from build123d import *

# Parameters (mm, degrees)
CROQUIS1_R              = 7.5
SALIENTE_EXTRUIR2_DEPTH = 20
SALIENTE_EXTRUIR3_DEPTH = 30
SALIENTE_EXTRUIR4_DEPTH = 80
CROQUIS4_R              = 10
CORTAR_EXTRUIR1_DEPTH   = 141.528466867


with BuildPart() as part:
    # Croquis1 → Saliente-Extruir2 (new body)
    # profile 1 of 7: a face of its own
    with BuildSketch(Plane(origin=(0, 0, 0), x_dir=(1, 0, 0), z_dir=(0, 1, 0))):
        with BuildLine():
            Line((74.169014085, 14.661423864), (6.338028169, 29.322847729))
            ThreePointArc((6.338028169, 29.322847729), (15.924993338, 25.424291282), (23.616731357, 18.5))
            ThreePointArc((23.616731357, 18.5), (26.900316488, 13.280548665), (29.047375097, 7.5))
            ThreePointArc((29.047375097, 7.5), (29.760890888, 3.780128774), (30, 0))
            ThreePointArc((30, 0), (29.760890888, -3.780128774), (29.047375097, -7.5))
            ThreePointArc((29.047375097, -7.5), (26.900316488, -13.280548665), (23.616731357, -18.5))
            ThreePointArc((23.616731357, -18.5), (15.924993338, -25.424291282), (6.338028169, -29.322847729))
            Line((6.338028169, -29.322847729), (74.169014085, -14.661423864))
            ThreePointArc((74.169014085, -14.661423864), (86, 0), (74.169014085, 14.661423864))
        make_face()
        with Locations(Location((71, 0, 0), (0, 0, 270))):
            Circle(CROQUIS1_R, mode=Mode.SUBTRACT)
    # profile 2 of 7: a face of its own
    with BuildSketch(Plane(origin=(0, 0, 0), x_dir=(1, 0, 0), z_dir=(0, 1, 0))):
        with BuildLine():
            ThreePointArc((-29.047375097, -7.5), (-26.900316488, -13.280548665), (-23.616731357, -18.5))
            Line((-23.616731357, -18.5), (23.616731357, -18.5))
            ThreePointArc((23.616731357, -18.5), (26.900316488, -13.280548665), (29.047375097, -7.5))
            Line((29.047375097, -7.5), (-29.047375097, -7.5))
        make_face()
    # profile 3 of 7: a face of its own
    with BuildSketch(Plane(origin=(0, 0, 0), x_dir=(1, 0, 0), z_dir=(0, 1, 0))):
        with BuildLine():
            ThreePointArc((-23.616731357, -18.5), (-15.924993338, -25.424291282), (-6.338028169, -29.322847729))
            ThreePointArc((-6.338028169, -29.322847729), (0, -30), (6.338028169, -29.322847729))
            ThreePointArc((6.338028169, -29.322847729), (15.924993338, -25.424291282), (23.616731357, -18.5))
            Line((23.616731357, -18.5), (-23.616731357, -18.5))
        make_face()
    # profile 4 of 7: a face of its own
    with BuildSketch(Plane(origin=(0, 0, 0), x_dir=(1, 0, 0), z_dir=(0, 1, 0))):
        with BuildLine():
            Line((29.047375097, 7.5), (-29.047375097, 7.5))
            ThreePointArc((-29.047375097, 7.5), (-30, 0), (-29.047375097, -7.5))
            Line((-29.047375097, -7.5), (29.047375097, -7.5))
            ThreePointArc((29.047375097, -7.5), (29.760890888, -3.780128774), (30, 0))
            ThreePointArc((30, 0), (29.760890888, 3.780128774), (29.047375097, 7.5))
        make_face()
    # profile 5 of 7: a face of its own
    with BuildSketch(Plane(origin=(0, 0, 0), x_dir=(1, 0, 0), z_dir=(0, 1, 0))):
        with BuildLine():
            Line((23.616731357, 18.5), (-23.616731357, 18.5))
            ThreePointArc((-23.616731357, 18.5), (-26.900316488, 13.280548665), (-29.047375097, 7.5))
            Line((-29.047375097, 7.5), (29.047375097, 7.5))
            ThreePointArc((29.047375097, 7.5), (26.900316488, 13.280548665), (23.616731357, 18.5))
        make_face()
    # profile 6 of 7: a face of its own
    with BuildSketch(Plane(origin=(0, 0, 0), x_dir=(1, 0, 0), z_dir=(0, 1, 0))):
        with BuildLine():
            ThreePointArc((6.338028169, 29.322847729), (0, 30), (-6.338028169, 29.322847729))
            ThreePointArc((-6.338028169, 29.322847729), (-15.924993338, 25.424291282), (-23.616731357, 18.5))
            Line((-23.616731357, 18.5), (23.616731357, 18.5))
            ThreePointArc((23.616731357, 18.5), (15.924993338, 25.424291282), (6.338028169, 29.322847729))
        make_face()
    # profile 7 of 7: a face of its own
    with BuildSketch(Plane(origin=(0, 0, 0), x_dir=(1, 0, 0), z_dir=(0, 1, 0))):
        with BuildLine():
            Line((-6.338028169, 29.322847729), (-74.169014085, 14.661423864))
            ThreePointArc((-74.169014085, 14.661423864), (-86, 0), (-74.169014085, -14.661423864))
            Line((-74.169014085, -14.661423864), (-6.338028169, -29.322847729))
            ThreePointArc((-6.338028169, -29.322847729), (-15.924993338, -25.424291282), (-23.616731357, -18.5))
            ThreePointArc((-23.616731357, -18.5), (-26.900316488, -13.280548665), (-29.047375097, -7.5))
            ThreePointArc((-29.047375097, -7.5), (-30, 0), (-29.047375097, 7.5))
            ThreePointArc((-29.047375097, 7.5), (-26.900316488, 13.280548665), (-23.616731357, 18.5))
            ThreePointArc((-23.616731357, 18.5), (-15.924993338, 25.424291282), (-6.338028169, 29.322847729))
        make_face()
        with Locations(Location((-71, 0, 0), (0, 0, 270))):
            Circle(CROQUIS1_R, mode=Mode.SUBTRACT)
    extrude(amount=SALIENTE_EXTRUIR2_DEPTH)

    # Croquis2 → Saliente-Extruir3 (add)
    with BuildSketch(Plane(origin=(0, 20, 0), x_dir=(1, 0, 0), z_dir=(0, 1, 0))):
        with BuildLine():
            Line((-23.616731357, 18.5), (23.616731357, 18.5))
            ThreePointArc((23.616731357, 18.5), (0, 30), (-23.616731357, 18.5))
        make_face()
        with BuildLine():
            Line((-23.616731357, -18.5), (23.616731357, -18.5))
            ThreePointArc((23.616731357, -18.5), (0, -30), (-23.616731357, -18.5))
        make_face()
    extrude(amount=SALIENTE_EXTRUIR3_DEPTH)

    # Croquis3 → Saliente-Extruir4 (add)
    with BuildSketch(Plane(origin=(0, 20, 0), x_dir=(1, 0, 0), z_dir=(0, 1, 0))):
        with BuildLine():
            ThreePointArc((-23.616731357, 18.5), (-26.900316488, 13.280548665), (-29.047375097, 7.5))
            Line((-29.047375097, 7.5), (29.047375097, 7.5))
            ThreePointArc((29.047375097, 7.5), (26.900316488, 13.280548665), (23.616731357, 18.5))
            Line((23.616731357, 18.5), (-23.616731357, 18.5))
        make_face()
        with BuildLine():
            Line((-29.047375097, -7.5), (29.047375097, -7.5))
            ThreePointArc((29.047375097, -7.5), (26.900316391, -13.280548617), (23.616731357, -18.5))
            Line((23.616731357, -18.5), (-23.616731357, -18.5))
            ThreePointArc((-23.616731357, -18.5), (-26.900316488, -13.280548665), (-29.047375097, -7.5))
        make_face()
    extrude(amount=SALIENTE_EXTRUIR4_DEPTH)

    # Croquis4 → Cortar-Extruir1 (cut, through all)
    with BuildSketch(Plane.XY.offset(18.5)):
        with Locations((0, 76)):
            Circle(CROQUIS4_R)
    extrude(amount=-CORTAR_EXTRUIR1_DEPTH, mode=Mode.SUBTRACT)


solid = part.part
Input: part model. Units: mm. Frame: model coordinates. A direction names the side the tool comes from. Coordinates: 2 decimals unless noted, no trailing zeros. Order: outer loops, then holes, each group sorted by start corner. A loop starts at its lowest first (then second) coordinate and runs counter-clockwise, first axis right, second up. Notation, with made-up numbers: M -31.75,-4.75 L 9.25,-4.75 A25 cw 9.25,19.25 Z; hole C -7,37 d3. An arc over 180 degrees is marked long. Answer in a Markdown table with one row per item.
(1) Section query C-C, the plane y = 40.5. Output: boundary loops of the cut face in (x, z).
Numbers:
| item | result |
|---|---|
| outline | M -29.05,-7.5 A30 ccw 29.05,-7.5 Z; M -29.05,7.5 L 29.05,7.5 A30 ccw 23.62,18.5 A30 ccw Z |
(2) Draft query along X for faces 1 (the cylindrical face through (-77.654, 9.86, 3.461)), 2 (the flat face through (39.779, 9.86, 22.095)), 3 (the cylindrical face through (63.68, 9.86, -1.63)), 4 (the flat face through (0, 50, -23)). Return one class per face: pulls with the +X half, pulls with the -X half, needs draft (parallel to the pull), parting line crosses it, or undercut.
Numbers:
| item | result |
|---|---|
| face 1 | undercut |
| face 2 | pulls with the +X half |
| face 3 | undercut |
| face 4 | needs draft |
(3) Access query for faces 5 (the flat face through (0, 50, 23)), 6 (the flat face through (0, 100, -13)), 7 (the flat face through (0, 59, -7.5)). Directions: +Z, -Z, +X, -X, +Y, -Y. A direction counts if a zero-diameter tool reaches every point of the face in a straight line with its end or side. Return the directions, or none.
Numbers:
| item | result |
|---|---|
| face 5 | +Z, +X, -X, +Y |
| face 6 | +Z, -Z, +X, -X, +Y |
| face 7 | +X, -X, +Y |
(4) Material intervals for line 1 (X direction, y = 15, z = 0); line 2 (Y direction, x = -76, z = -6); line 3 (Z direction, x = -1, y = 30), sorted ascending. Write a range as [from, to].
Numbers:
| item | result |
|---|---|
| line 1 | x = [-86, -78.5], [-63.5, 63.5], [78.5, 86] |
| line 2 | y = [0, 20] |
| line 3 | z = [-29.98, -7.5], [7.5, 29.98] |
(5) Section query D-D, the plane x = 3.5. Output: boundary loops of the cut face in (y, z).
Numbers:
| item | result |
|---|---|
| outline | M 0,-29.8 L 50,-29.8 L 50,-18.5 L 66.63,-18.5 L 66.63,-7.5 L 20,-7.5 L 20,7.5 L 66.63,7.5 L 66.63,18.5 L 50,18.5 L 50,29.8 L 0,29.8 Z; M 85.37,-18.5 L 100,-18.5 L 100,-7.5 L 85.37,-7.5 Z; M 85.37,7.5 L 100,7.5 L 100,18.5 L 85.37,18.5 Z |
(6) Section query B-B, the plane y = 76. Output: boundary loops of the cut face in (x, z), plus the area to 3 significant figures.
Numbers:
| item | result |
|---|---|
| outline | M -29.05,-7.5 A30 ccw -23.62,-18.5 L -10,-18.5 L -10,-7.5 Z; M -29.05,7.5 L -10,7.5 L -10,18.5 L -23.62,18.5 A30 ccw Z; M 10,-18.5 L 23.62,-18.5 A30 ccw 29.05,-7.5 L 10,-7.5 Z; M 10,7.5 L 29.05,7.5 A30 ccw 23.62,18.5 L 10,18.5 Z |
| area | 739 mm^2 |
(7) Contact query for flat-ended pins moving along their axis: pin 1 Ø6 at (y, z) = (86, -16.5) entering from -X; pin 2 Ø4 at (y, z) = (73.5, 8.5) entering from -X; pin 3 Ø12 at (x, y) = (0, 76) entering from -Z; pin 4 Ø6 at (x, z) = (-10.5, 27) entering from +Y. Output: stop coordinate, or through.
Numbers:
| item | result |
|---|---|
| pin 1 | stops at x = -26.79 |
| pin 2 | stops at x = -29.05 |
| pin 3 | passes through |
| pin 4 | stops at y = 50 |
(8) Section query A-A, the plane z = 0. Output: boundary loops of the cut face in (x, y).
Numbers:
| item | result |
|---|---|
| outline | M -86,0 L -78.5,0 L -78.5,20 L -86,20 Z; M -63.5,0 L 63.5,0 L 63.5,20 L -63.5,20 Z; M 78.5,0 L 86,0 L 86,20 L 78.5,20 Z |
